For this review, take the finished solid that the model builds, in its own axes (mm). Face numbers are marked on the shaded views. A direction names the side the tool comes from. Give positions to 0.01 mm unless a question says otherwise; leave off trailing zeros. Write each loop counter-clockwise with the first axis right and the second up, starting at its lowest first coordinate (ties: lowest second). Pieces come first, ordered by that corner, then holes. Notation, with made-up numbers: (-5, 27.25) -> (51, 27.25) arc R14 ccw to (51, 39.25) -> close; hole circle Ø3 at (50, 74). An arc over 180 degrees is marked (long way). Answer as CSV lines item,"result".
Autodesk Inventor part; units mm, degrees
ref_plane "YZ Plane" through (0, 0, 0) normal (1, 0, 0) x (0, 1, 0)
ref_plane "XZ Plane" through (0, 0, 0) normal (0, 1, 0) x (-1, 0, 0)
ref_plane "XY Plane" through (0, 0, 0) normal (0, 0, 1) x (1, 0, 0)
sketch "Sketch1" plane through (0, 0, 0) normal (0, 1, 0) x (-1, 0, 0)
  line L0 (17.5, 17.8107) -> (17.5, 41.4147) construction
  line L1 (35, 60.5) -> (35, 0)
  line L2 (30, 17.5) -> (30, 26)
  line L3 (30, 26) -> (29, 26)
  line L4 (29, 26) -> (29, 17.5)
  line L5 (29, 17.5) -> (30, 17.5)
  line L6 (29, 34.5) -> (30, 34.5)
  line L7 (30, 34.5) -> (30, 43)
  line L8 (30, 43) -> (29, 43)
  line L9 (29, 43) -> (29, 34.5)
  line L10 (30, 57.75) -> (30, 60.5)
  line L11 (30, 60.5) -> (35, 60.5)
  line L12 (10, 57.75) -> (10, 60.5)
  line L13 (30, 57.75) -> (10, 57.75)
  line L14 (30, 2.75) -> (30, 0)
  line L15 (30, 0) -> (35, 0)
  line L16 (10, 2.75) -> (10, 0)
  line L17 (30, 2.75) -> (10, 2.75)
  line L18 (0, 50.75) -> (-2.75, 50.75)
  line L19 (-2.75, 50.75) -> (-2.75, 43.75)
  line L20 (-2.75, 43.75) -> (0, 43.75)
  line L21 (0, 16.75) -> (-2.75, 16.75)
  line L22 (-2.75, 16.75) -> (-2.75, 9.75)
  line L23 (-2.75, 9.75) -> (0, 9.75)
  line L24 (17.3275, 30.25) -> (11.5049, 30.25) construction
  line L25 (0, 50.75) -> (0, 57.75)
  line L26 (0, 2.75) -> (0, 9.75)
  line L27 (0, 16.75) -> (0, 43.75)
  line L28 (10, 0) -> (5, 0)
  line L29 (5, 0) -> (5, 2.75)
  line L30 (5, 2.75) -> (0, 2.75)
  line L31 (10, 60.5) -> (5, 60.5)
  line L32 (5, 60.5) -> (5, 57.75)
  line L33 (5, 57.75) -> (0, 57.75)
  point P0 (0, 0)
  point P1 (0, 0)
  point P2 (0, 0)
  point P3 (0, 0)
  point P4 (0, 0)
  point P5 (30.5, 47.25)
  point P6 (30.5, 30.25)
  point P7 (30.5, 13.25)
  dimension "d151" = 8.5
  dimension "d153" = 1
  dimension "d155" = 5
  dimension "d159" = 17
  dimension "d160" = 17
  dimension "d161" = 4.25
  dimension "d162" = 4.25
  dimension "d176" = 4.5
  dimension "d177" = 5
  dimension "d179" = 55
  dimension "d180" = 2.75
  dimension "d182" = 7
  dimension "d183" = 7
  dimension "d184" = 35
extrude "Extrusion1" add sketch "Sketch1" against normal blind 1.5
hole "Hole1" at (-30.5, 0, 47.25) at (-30.5, 0, 30.25) at (-30.5, 0, 13.25) direction (0, -1, 0) diameter 1 end through all
sketch "Sketch4" plane through (0, 0, 0) normal (0, 1, 0) x (1, 0, 0)
  line L0 (-3, -46.55) -> (-3, -3.25)
  line L1 (-3, -3.25) -> (-21, -3.25)
  line L2 (-21, -3.25) -> (-21, -46.55)
  line L3 (-21, -46.55) -> (-3, -46.55)
  line L4 (-30, -2.75) -> (-10, -2.75)
  line L5 (-10, -2.75) -> (-30, -2.75)
  line L6 (0, -43.75) -> (0, -16.75)
  point P0 (0, 0)
  dimension "d188" = 43.3
  dimension "d189" = 18
  dimension "d190" = 3
  dimension "d212" = 0.5
extrude "Extrusion11" add sketch "Sketch4" along normal blind 5
sketch "Sketch6" plane through (0, 5, 0) normal (0, 1, 0) x (1, 0, 0)
  line L0 (-17.0504, -18.7342) -> (-12.1007, -13.7844)
  line L1 (-12.1007, -13.7844) -> (-7.1509, -18.7342)
  line L2 (-7.1509, -18.7342) -> (-12.1007, -23.6839)
  line L3 (-12.1007, -23.6839) -> (-17.0504, -18.7342)
  point P0 (0, 0)
  dimension "d198" = 7
  dimension "d199" = 7
extrude "Extrusion13" add sketch "Sketch6" along normal blind 2
sketch "Sketch7" plane through (0, 5, 0) normal (0, 1, 0) x (1, 0, 0)
  line L0 (-15.6959, -40.3292) -> (-8.6959, -40.3292)
  line L1 (-8.6959, -40.3292) -> (-8.6959, -45.3292)
  line L2 (-8.6959, -45.3292) -> (-15.6959, -45.3292)
  line L3 (-15.6959, -45.3292) -> (-15.6959, -40.3292)
  point P0 (0, 0)
  dimension "d202" = 7
  dimension "d203" = 5
extrude "Extrusion14" add sketch "Sketch7" along normal blind 2.5
sketch "Sketch8" plane through (0, 7.5, 0) normal (0, 1, 0) x (1, 0, 0)
  line L0 (-15.3142, -41.2282) -> (-14.6142, -41.2282)
  line L1 (-14.6142, -41.2282) -> (-14.6142, -41.9282)
  line L2 (-14.6142, -41.9282) -> (-15.3142, -41.9282)
  line L3 (-15.3142, -41.9282) -> (-15.3142, -41.2282)
  line L4 (-15.3142, -43.9282) -> (-14.6142, -43.9282)
  line L5 (-14.6142, -43.9282) -> (-14.6142, -44.6282)
  line L6 (-14.6142, -44.6282) -> (-15.3142, -44.6282)
  line L7 (-15.3142, -44.6282) -> (-15.3142, -43.9282)
  line L8 (-12.6142, -41.2282) -> (-11.9142, -41.2282)
  line L9 (-11.9142, -41.2282) -> (-11.9142, -41.9282)
  line L10 (-11.9142, -41.9282) -> (-12.6142, -41.9282)
  line L11 (-12.6142, -41.9282) -> (-12.6142, -41.2282)
  line L12 (-12.6142, -43.9282) -> (-11.9142, -43.9282)
  line L13 (-11.9142, -43.9282) -> (-11.9142, -44.6282)
  line L14 (-11.9142, -44.6282) -> (-12.6142, -44.6282)
  line L15 (-12.6142, -44.6282) -> (-12.6142, -43.9282)
  line L16 (-9.9142, -41.2282) -> (-9.2142, -41.2282)
  line L17 (-9.2142, -41.2282) -> (-9.2142, -41.9282)
  line L18 (-9.2142, -41.9282) -> (-9.9142, -41.9282)
  line L19 (-9.9142, -41.9282) -> (-9.9142, -41.2282)
  line L20 (-9.9142, -43.9282) -> (-9.2142, -43.9282)
  line L21 (-9.2142, -43.9282) -> (-9.2142, -44.6282)
  line L22 (-9.2142, -44.6282) -> (-9.9142, -44.6282)
  line L23 (-9.9142, -44.6282) -> (-9.9142, -43.9282)
  point P0 (0, 0)
  dimension "d206" = 0.7
  dimension "d207" = 2
  dimension "d208" = 2
  dimension "d209" = 2
extrude "Extrusion15" add sketch "Sketch8" along normal blind 5
sketch "Sketch9" plane through (-3, 0, 3.25) normal (0, 0, -1) x (-1, 0, 0)
  line L0 (12.75, 8.5) -> (5.25, 8.5)
  line L1 (5.25, 8.5) -> (5.25, 5)
  line L2 (5.25, 5) -> (12.75, 5)
  line L3 (12.75, 5) -> (12.75, 8.5)
  line L4 (9, 5.7242) -> (9, 7.4058) construction
  line L5 (18, 0) -> (18, 5)
  line L6 (0, 5) -> (18, 5)
  point P0 (-3, 0)
  dimension "d213" = 7.5
  dimension "d214" = 3.5
  dimension "d215" = 9
extrude "Extrusion16" add sketch "Sketch9" along normal blind 2 and the other way blind 7
sketch "Sketch15" plane through (-3, 0, 1.25) normal (0, 0, -1) x (-1, 0, 0)
  line L0 (12.25, 8.25) -> (5.75, 8.25)
  line L1 (5.75, 8.25) -> (5.75, 5.25)
  line L2 (5.75, 5.25) -> (12.25, 5.25)
  line L3 (12.25, 5.25) -> (12.25, 8.25)
  line L4 (5.25, 8.5) -> (5.25, 5)
  line L5 (12.75, 8.5) -> (5.25, 8.5)
  point P0 (-3, 0)
  dimension "d242" = 6.5
  dimension "d243" = 3
  dimension "d244" = 0.5
  dimension "d245" = 0.25
extrude "Extrusion20" cut sketch "Sketch15" against normal blind 5
properties part number "Microcontroller_board_Nano_square" material "ABS Plastic"
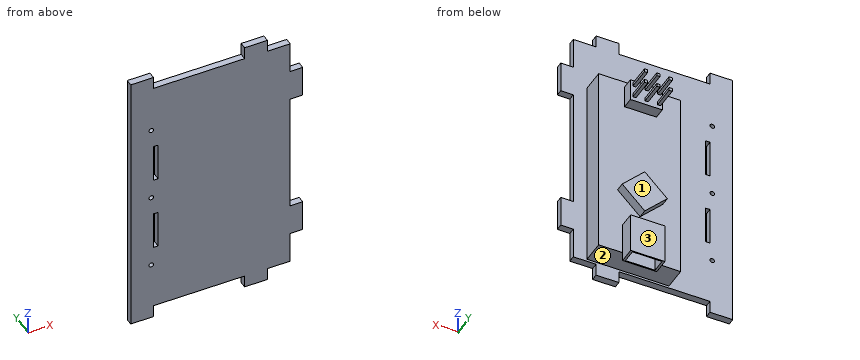
Q1. Add section C-C (z = 11). Write out the cut boundary in (x, y).
Answer block:
outline,"(-35, -1.5) -> (2.75, -1.5) -> (2.75, 0) -> (-3, 0) -> (-3, 5) -> (-21, 5) -> (-21, 0) -> (-35, 0) -> close"
Q2. Clearance check with flat-ended pins moving along their axes: pin 1 (4 mm diameter, centred on x = -13.5, z = 2.5, fed in from +Y); pin 2 (0.8 mm diameter, centred on y = -0.5, z = 2, fed in from +X); pin 3 (6 mm diameter, centred on x = -8, y = 6.5, fed in from +Z); pin 4 (6 mm diameter, centred on x = -30, y = 2, fed in from -Z). State where each tip first meets the part, or that it passes through.
Answer block:
pin 1,"stops at y = 8.5"
pin 2,"stops at x = -5"
pin 3,"stops at z = 46.55"
pin 4,"stops at z = 0"
Q3. Add section D-D (y = 2). Write out the cut boundary in (x, z).
Answer block:
outline,"(-21, 3.25) -> (-3, 3.25) -> (-3, 46.55) -> (-21, 46.55) -> close"
Q4. Add section B-B (y = 9.5). Write out the cut boundary in (x, z).
Answer block:
outline,"(-15.31, 41.23) -> (-14.61, 41.23) -> (-14.61, 41.93) -> (-15.31, 41.93) -> close; (-15.31, 43.93) -> (-14.61, 43.93) -> (-14.61, 44.63) -> (-15.31, 44.63) -> close; (-12.61, 41.23) -> (-11.91, 41.23) -> (-11.91, 41.93) -> (-12.61, 41.93) -> close; (-12.61, 43.93) -> (-11.91, 43.93) -> (-11.91, 44.63) -> (-12.61, 44.63) -> close; (-9.91, 41.23) -> (-9.21, 41.23) -> (-9.21, 41.93) -> (-9.91, 41.93) -> close; (-9.91, 43.93) -> (-9.21, 43.93) -> (-9.21, 44.63) -> (-9.91, 44.63) -> close"
Q5. To check wall thickness, follow probe 1 along Z at (x, y) = (-30.5, -1.2); probe 2 along X at (y, z) = (-0.8, 13.25); probe 3 along X at (y, z) = (6.75, 2.5). State the ranges of each line that lie inside material, in increasing order. Write a range as [from, to].
Answer block:
probe 1,"z = [0, 12.75], [13.75, 29.75], [30.75, 46.75], [47.75, 60.5]"
probe 2,"x = [-35, -31], [-30, 2.75]"
probe 3,"x = [-15.75, -15.25], [-8.75, -8.25]"
Q6. For the marked faces 1, 2 and 3, list the 3-axis set-ups (+Z, -Z, +X, -X, +Y, -Y) from which the entire face can be reached by the end or side of a thin tool; tool diameter is ignored.
Answer block:
face 1,"+X, -X, +Y"
face 2,"-Z, +X, -X"
face 3,"-Z, +X, -X, +Y"
Q7. Add section A-A (z = 38.5). Write out the cut boundary in (x, y).
Answer block:
outline,"(-35, -1.5) -> (-30, -1.5) -> (-30, 0) -> (-35, 0) -> close; (-29, -1.5) -> (0, -1.5) -> (0, 0) -> (-3, 0) -> (-3, 5) -> (-21, 5) -> (-21, 0) -> (-29, 0) -> close"
